For this review, take the finished solid that the model builds, in its own axes (mm). Round coordinates to 2 decimals unless told otherwise and drop trailing zeros. Order: outer loops, then holes, each group sorted by start corner. A loop starts at its lowest first (then second) coordinate and runs counter-clockwise, first axis right, second up. Notation, with made-up numbers: (-7, 64.25) - (1, 64.25) arc R19 ccw to (1, 84.25) - close; hole circle Ø11 at (59.25, 81). An arc over 180 degrees is marked (long way). Write each question's results on one line, items separated by ' | '. Start each with the question number.
(1) Take a section at A-A, the plane x = 14. Give the boundary of the cut face in (y, z) (3 decimals), plus the area to 3 significant figures.
(2) For L1, parallel to X at y = 43, z = 2.15; L2, parallel to Y at x = -19.5, z = 1.45, list the stretches that pass through material, from the lowest coordinate up. Write a range as from..to.
(3) Insertion check: pin 1 Ø1.6 at (x, z) = (83.5, 2) entering from -Y; pin 2 Ø1 at (y, z) = (83, 2.5) entering from +X; pin 3 Ø1 at (x, z) = (-20.5, 2) entering from -Y. Each pin has a flat end and moves straight along its axis. Give the tip position at first contact, or say it passes through.
(4) Take a section at B-B, the plane y = -56. Give the boundary of the cut face in (x, z) (3 decimals), plus the area to 3 significant figures.
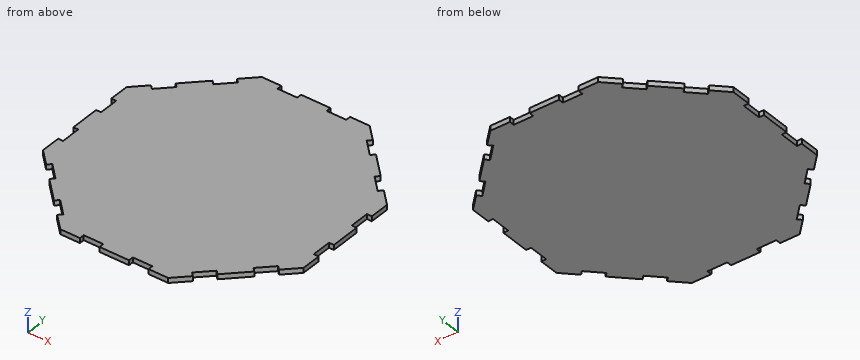
```python
from build123d import *

# Parameters (mm, degrees)
BOSS_EXTRUDE1_DEPTH = 3.175


with BuildPart() as part:
    # Sketch1 → Boss-Extrude1 (new body)
    with BuildSketch(Plane.XY):
        Polygon((50.640448212, 64.110832393), (41.660192091, 73.091088515), (43.905256121, 75.336152545), (34.925, 84.316408666), (22.225, 84.316408666), (22.225, 81.141408666), (9.525, 81.141408666), (9.525, 84.316408666), (-9.525, 84.316408666), (-9.525, 81.141408666), (-22.225, 81.141408666), (-22.225, 84.316408666), (-34.925, 84.316408666), (-43.905256121, 75.336152545), (-41.660192091, 73.091088515), (-50.640448212, 64.110832393), (-52.885512242, 66.355896424), (-66.355896424, 52.885512242), (-64.110832393, 50.640448212), (-73.091088515, 41.660192091), (-75.336152545, 43.905256121), (-84.316408666, 34.925), (-84.316408666, 22.225), (-81.141408666, 22.225), (-81.141408666, 9.525), (-84.316408666, 9.525), (-84.316408666, -9.525), (-81.141408666, -9.525), (-81.141408666, -22.225), (-84.316408666, -22.225), (-84.316408666, -34.925), (-75.336152545, -43.905256121), (-73.091088515, -41.660192091), (-64.110832393, -50.640448212), (-66.355896424, -52.885512242), (-52.885512242, -66.355896424), (-50.640448212, -64.110832393), (-41.660192091, -73.091088515), (-43.905256121, -75.336152545), (-34.925, -84.316408666), (-22.225, -84.316408666), (-22.225, -81.141408666), (-9.525, -81.141408666), (-9.525, -84.316408666), (9.525, -84.316408666), (9.525, -81.141408666), (22.225, -81.141408666), (22.225, -84.316408666), (34.925, -84.316408666), (43.905256121, -75.336152545), (41.660192091, -73.091088515), (50.640448212, -64.110832393), (52.885512242, -66.355896424), (66.355896424, -52.885512242), (64.110832393, -50.640448212), (73.091088515, -41.660192091), (75.336152545, -43.905256121), (84.316408666, -34.925), (84.316408666, -22.225), (81.141408666, -22.225), (81.141408666, -9.525), (84.316408666, -9.525), (84.316408666, 9.525), (81.141408666, 9.525), (81.141408666, 22.225), (84.316408666, 22.225), (84.316408666, 34.925), (75.336152545, 43.905256121), (73.091088515, 41.660192091), (64.110832393, 50.640448212), (66.355896424, 52.885512242), (52.885512242, 66.355896424), align=None)
    extrude(amount=BOSS_EXTRUDE1_DEPTH)


solid = part.part
```
Results below:
1) outline: (-81.141, 0) - (81.141, 0) - (81.141, 3.175) - (-81.141, 3.175) - close | area: 515 mm^2
2) L1: x = -76.24..-74.43, -71.75..71.75, 74.43..76.24 | L2: y = -81.14..81.14
3) pin 1: stops at y = -36.54 | pin 2: stops at x = 36.74 | pin 3: stops at y = -81.14
4) outline: (-63.241, 0) - (63.241, 0) - (63.241, 3.175) - (-63.241, 3.175) - close | area: 402 mm^2
